Input: part model. Units: mm. Frame: model coordinates. A direction names the side the tool comes from. Give positions to 0.01 mm unless a question says otherwise; leave off trailing zeros. Order: outer loops, then holes, each group sorted by start corner. A loop starts at its lowest first (then second) coordinate and runs counter-clockwise, first axis right, second up. Notation, with made-up numbers: (-24, -21.75) -> (-11, -21.75) arc R19 cw to (-11, 1.25) -> close; hole circle Ø7 at (52, 40.25). An arc over 180 degrees is marked (long way). Use a Markdown table: item, result. Add a question column.
Solid Edge part; units mm, degrees
sketch "Sketch1" plane through (0, 0, 0) normal (1, 0, 0) x (0, 1, 0)
  circle A0 centre (0, 0) radius 4
  circle A1 centre (0, 0) radius 25
extrude "Protrusion1" add sketch "Sketch1" along normal blind 8
sketch "Sketch2" plane through (0, 0, 0) normal (-1, 0, 0) x (0, -1, 0)
  circle A0 centre (0, 0) radius 6.45
extrude "ExtrudedCutout_1" cut sketch "Sketch2" against normal blind 5.8
sketch "Sketch3" plane through (8, 0, 0) normal (1, 0, 0) x (0, 1, 0)
  circle A0 centre (-22, 0) radius 1.6
extrude "Cutout1" cut sketch "Sketch3" against normal up to next
pattern_circular "Pattern1" count 6 over 360 about axis through (8, 0, 0) along (-1, 0, 0) of "Cutout1"
Q1. Section query A-A (y = 0). Return loops of the section in (x, z), plus the area to 3 significant figures.
Q2. Section query C-C (y = 11). Return loops of the section in (x, z).
Q3. First-contact query: pin 1 (2 mm diameter, centred on x = 3.5, z = -18, fed in from +Y); pin 2 (1.5 mm diameter, centred on x = 1.5, z = -3, fed in from +Y). Flat tips, straight axial feed; report the tip coordinate or a pass-through.
Q4. Draft query along Y for faces 3 (the cylindrical face through (3.944, 23.846, -7.509)), 4 (the cylindrical face through (4.06, -9.73, -18.08)), 5 (the flat face through (0, 5, 5)). Return one class per face: +Y half, -Y half, draft (parallel to the pull), parting line (faces both ways), or undercut.
Q5. Access query for faces 1 (the cylindrical face through (4.06, 9.73, 18.08)), 2 (the cylindrical face through (2.859, 1.398, -6.297)). Directions: +Z, -Z, +X, -X, +Y, -Y. A direction counts if a zero-diameter tool reaches every point of the face in a straight line with its end or side. Return the directions, or none.
Q6. Section query B-B (z = 0). Return loops of the section in (x, y), plus the area to 3 significant figures.
Q7. Ray query, line 1 (Z direction, x = 4, y = 11); line 2 (Z direction, x = 1.75, y = 22); line 3 (Z direction, x = 7.25, y = 0). Return the intervals inside material, ascending.
Q8. Section query D-D (x = 2.5). Return loops of the section in (y, z), plus the area to 3 significant figures.
Solution:
| question | item | result |
|---|---|---|
| 1 | outline | (0, -25) -> (8, -25) -> (8, -4) -> (5.8, -4) -> (5.8, -6.45) -> (0, -6.45) -> close; (0, 6.45) -> (5.8, 6.45) -> (5.8, 4) -> (8, 4) -> (8, 25) -> (0, 25) -> close |
| 1 | area | 308 mm² |
| 2 | outline | (0, -22.45) -> (8, -22.45) -> (8, -20.65) -> (0, -20.65) -> close; (0, -17.45) -> (8, -17.45) -> (8, 17.45) -> (0, 17.45) -> close; (0, 20.65) -> (8, 20.65) -> (8, 22.45) -> (0, 22.45) -> close |
| 3 | pin 1 | stops at y = 18.33 |
| 3 | pin 2 | stops at y = 24.9 |
| 4 | face 3 | parting line |
| 4 | face 4 | undercut |
| 4 | face 5 | draft |
| 5 | face 1 | +X, -X |
| 5 | face 2 | -X |
| 6 | outline | (0, -25) -> (8, -25) -> (8, -23.6) -> (0, -23.6) -> close; (0, -20.4) -> (8, -20.4) -> (8, -4) -> (5.8, -4) -> (5.8, -6.45) -> (0, -6.45) -> close; (0, 6.45) -> (5.8, 6.45) -> (5.8, 4) -> (8, 4) -> (8, 20.4) -> (0, 20.4) -> close; (0, 23.6) -> (8, 23.6) -> (8, 25) -> (0, 25) -> close |
| 6 | area | 256 mm² |
| 7 | line 1 | z = -22.45 to -20.65, -17.45 to 17.45, 20.65 to 22.45 |
| 7 | line 2 | z = -11.87 to -1.6, 1.6 to 11.87 |
| 7 | line 3 | z = -25 to -4, 4 to 25 |
| 8 | outline | circle Ø50 at (0, 0); hole circle Ø3.2 at (-22, 0); hole circle Ø3.2 at (-11, -19.05); hole circle Ø3.2 at (-11, 19.05); hole circle Ø12.9 at (0, 0); hole circle Ø3.2 at (11, -19.05); hole circle Ø3.2 at (11, 19.05); hole circle Ø3.2 at (22, 0) |
| 8 | area | 1,780 mm² |
